Check sheet for the modelled part. Datum: model origin and axes. Units: mm. A direction names the side the tool comes from. Give positions to 0.01 mm unless a question says otherwise; leave off trailing zeros. Order: outer loops, then holes, each group sorted by start corner. A loop starts at its lowest first (then second) coordinate and runs counter-clockwise, first axis right, second up. Notation, with made-up numbers: (9.25, 46.25) -> (39.25, 46.25) arc R27 ccw to (39.25, 75.25) -> close; hole circle Ø9 at (49.5, 4.5). An arc over 180 degrees is marked (long way). Answer in a Markdown table with one row per item. Add a question column.
(1) Go/stop test with flat-tipped pins: pin 1 (8 mm diameter, centred on y = -69, z = 11, fed in from +X); pin 2 (1 mm diameter, centred on y = -49, z = 18, fed in from +X); pin 3 (22.5 mm diameter, centred on x = -8.5, y = -41.5, fed in from +Z); pin 4 (6 mm diameter, centred on x = 4.5, y = -82, fed in from +Z). Record where each tip stops, or that it passes through.
(2) Release check for a two-part mould opening along X. For faces 3 (the face through (-10.081, -103.015, 10.367)), 4 (the face through (-33.667, -30.004, 10.14)), 5 (the face through (-10.099, -104.014, 9.86)) record: released by +X, released by -X, zero draft, split by the parting line, or undercut.
(3) Cross-section at A-A (z = 2.75). Record the cut outline in (x, y).
(4) Cross-section at C-C (y = -12). Record the cut outline in (x, z).
(5) Set-up check for faces 1 (the face through (-23.54, -65.14, 10.37)), 2 (the face through (-24.503, -65.401, 9.86)): record each of +Z, -Z, +X, -X, +Y, -Y from which the full face is reachable in a straight line by a thin tool's end or side.
(6) Cross-section at B-B (x = -10). Record the cut outline in (y, z).
(7) Cross-section at D-D (z = 14). Record the cut outline in (x, y).
(8) Thickness scan on L1, parallel to Y at x = -10, z = 0.3; L2, parallel to Z at x = -8, y = -67; L3, parallel to Y at x = -11, z = 12.75. Record the ranges inside material, lowest first. Write a range as [from, to].
```python
from build123d import *

# Parameters (mm, degrees)
EXTRUDE_1_DEPTH     = 20
FILLET_1_R          = 5
SHELL_1_T           = -1
SKETCH_2_R          = 5
CUT_EXTRUDE_1_DEPTH = 20
CUT_EXTRUDE_2_REACH = 116.219
SKETCH_3_W          = 10
SKETCH_3_H          = 20


with BuildPart() as part:
    # 草图1 → 凸台-拉伸1 (new body)
    with BuildSketch(Plane.XY):
        with BuildLine():
            Line((0, 0), (-20, 0))
            Line((-20, 0), (-33.989229745, -30))
            Line((-33.989229745, -30), (-15.232786274, -100))
            ThreePointArc((-15.232786274, -100), (-10, -104.015258131), (-4.767213726, -100))
            Line((-4.767213726, -100), (13.989229745, -30))
            Line((13.989229745, -30), (0, 0))
        make_face()
    extrude(amount=EXTRUDE_1_DEPTH)

    # 圆角1
    fillet_1_edges = [part.edges().sort_by_distance(p)[0] for p in [
        (13.989229745, -30, 10),
        (-33.989229745, -30, 10),
        (-20, 0, 10),
        (0, 0, 10),
    ]]
    fillet(fillet_1_edges, radius=FILLET_1_R)

    # 抽壳1
    shell_1_openings = [part.faces().sort_by_distance(p)[0] for p in [
        (-10, -44.685846185, 20),
    ]]
    offset(amount=SHELL_1_T, openings=shell_1_openings, kind=Kind.INTERSECTION)

    # 草图2 → 切除-拉伸1 (cut)
    with BuildSketch(Plane(origin=(0, 0, 0), x_dir=(-1, 0, 0), z_dir=(0, 0, -1))):
        with Locations((10, -12)):
            Circle(SKETCH_2_R)
    extrude(amount=-CUT_EXTRUDE_1_DEPTH, mode=Mode.SUBTRACT)

    # 草图3 → 切除-拉伸2 (cut, up to next)
    with BuildSketch(Plane(origin=(20.552129041, -5.506926379, 0), x_dir=(0, 0, -1), z_dir=(0.9659258262890672, -0.2588190451025249, 0)), mode=Mode.PRIVATE) as cut_extrude_2_sk1:
        with Locations((-10, -81.826428333)):
            Rectangle(SKETCH_3_W, SKETCH_3_H)
    cut_extrude_2_tool1 = extrude(cut_extrude_2_sk1.sketch, amount=-CUT_EXTRUDE_2_REACH, mode=Mode.PRIVATE) & part.part
    add(cut_extrude_2_tool1.solids().sort_by_distance((-0.626109, -84.545187, 10))[0], mode=Mode.SUBTRACT)


solid = part.part
```
Answer below:
| question | item | result |
|---|---|---|
| 1 | pin 1 | stops at x = 4.61 |
| 1 | pin 2 | stops at x = 9.03 |
| 1 | pin 3 | stops at z = 1 |
| 1 | pin 4 | passes through |
| 2 | face 3 | undercut |
| 2 | face 4 | released by -X |
| 2 | face 5 | split by the parting line |
| 3 | outline | (-33.52, -31.76) -> (-15.23, -100) arc R5.42 ccw to (-4.77, -100) -> (13.52, -31.76) arc R5 ccw to (13.22, -28.35) -> (1.35, -2.89) arc R5 ccw to (-3.19, 0) -> (-16.81, 0) arc R5 ccw to (-21.35, -2.89) -> (-33.22, -28.35) arc R5 ccw to start; hole (-32.55, -31.5) -> (-14.27, -99.74) arc R4.42 ccw to (-5.73, -99.74) -> (12.55, -31.5) arc R4 ccw to (12.31, -28.77) -> (0.44, -3.31) arc R4 ccw to (-3.19, -1) -> (-16.81, -1) arc R4 ccw to (-20.44, -3.31) -> (-32.31, -28.77) arc R4 ccw to start |
| 4 | outline | (-25.6, 0) -> (-15, 0) -> (-15, 1) -> (-24.49, 1) -> (-24.49, 20) -> (-25.6, 20) -> close; (-5, 0) -> (5.6, 0) -> (5.6, 20) -> (4.49, 20) -> (4.49, 1) -> (-5, 1) -> close |
| 5 | face 1 | +Z |
| 5 | face 2 | +Z, -Z, -X, -Y |
| 6 | outline | (-104.02, 0) -> (-17, 0) -> (-17, 1) -> (-103.02, 1) -> (-103.02, 20) -> (-104.02, 20) -> close; (-7, 0) -> (0, 0) -> (0, 20) -> (-1, 20) -> (-1, 1) -> (-7, 1) -> close |
| 7 | outline | (-33.52, -31.76) -> (-15.23, -100) arc R5.42 ccw to (-4.77, -100) -> (-3.21, -94.2) -> (-4.18, -93.95) -> (-5.73, -99.74) arc R4.42 cw to (-14.27, -99.74) -> (-32.55, -31.5) arc R4 cw to (-32.31, -28.77) -> (-20.44, -3.31) arc R4 cw to (-16.81, -1) -> (-3.19, -1) arc R4 cw to (0.44, -3.31) -> (12.31, -28.77) arc R4 cw to (12.55, -31.5) -> (1, -74.63) -> (1.96, -74.89) -> (13.52, -31.76) arc R5 ccw to (13.22, -28.35) -> (1.35, -2.89) arc R5 ccw to (-3.19, 0) -> (-16.81, 0) arc R5 ccw to (-21.35, -2.89) -> (-33.22, -28.35) arc R5 ccw to start |
| 8 | L1 | y = [-104.02, -17], [-7, 0] |
| 8 | L2 | z = [0, 1] |
| 8 | L3 | y = [-103.92, -102.9], [-1, 0] |
